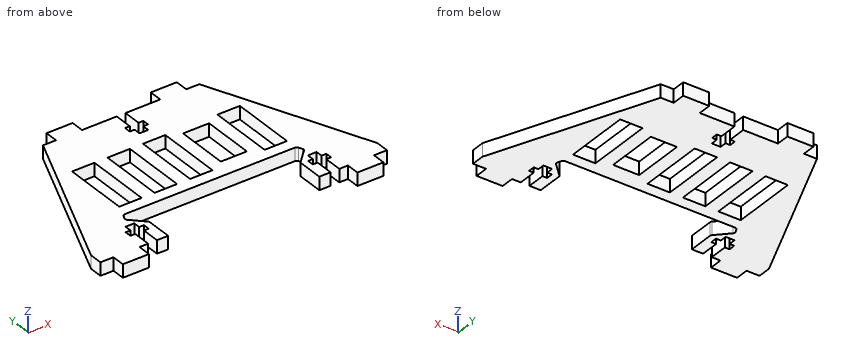
```python
from build123d import *

# Parameters (mm, degrees)
SKETCH1_W               = 139.7
SKETCH1_H               = 82.55
BOSS_EXTRUDE1_DEPTH     = 6.35
SKETCH2_W               = 12.7
SKETCH2_H               = 6.35
BOSS_EXTRUDE2_DEPTH     = 6.35
CUT_EXTRUDE1_DEPTH      = 6.35
CUT_EXTRUDE8_DEPTH      = 6.35
CUT_EXTRUDE2_DEPTH      = 6.35
CUT_EXTRUDE9_DEPTH      = 85.77904001
CUT_EXTRUDE9_DEPTH_BACK = 85.77904001
FILLET1_R               = 1.27
SKETCH9_W               = 10.922
SKETCH9_H               = 31.75
SKETCH9_W_2             = 12.7
SKETCH9_H_2             = 25.4
CUT_EXTRUDE10_DEPTH     = 6.35


with BuildPart() as part:
    # Sketch1 → Boss-Extrude1 (new body)
    with BuildSketch(Plane.XY):
        Rectangle(SKETCH1_W, SKETCH1_H)
    extrude(amount=BOSS_EXTRUDE1_DEPTH)

    # Sketch2 → Boss-Extrude2 (add)
    with BuildSketch(Plane(origin=(0, 0, 0), x_dir=(-1, 0, 0), z_dir=(0, 0, -1))):
        with Locations((-57.15, -44.45)):
            Rectangle(SKETCH2_W, SKETCH2_H)
        with Locations((-25.4, 44.45)):
            Rectangle(SKETCH2_W, SKETCH2_H)
    boss_extrude2 = extrude(amount=-BOSS_EXTRUDE2_DEPTH)

    # Sketch3 → Cut-Extrude1 (cut)
    with BuildSketch(Plane(origin=(0, 0, 0), x_dir=(-1, 0, 0), z_dir=(0, 0, -1))):
        Polygon((-46.5836, -41.275), (-46.5836, -32.512), (-48.895, -32.512), (-48.895, -29.337), (-46.5836, -29.337), (-46.5836, -26.035), (-42.3164, -26.035), (-42.3164, -29.337), (-40.005, -29.337), (-40.005, -32.512), (-42.3164, -32.512), (-42.3164, -41.275), align=None)
    cut_extrude1 = extrude(amount=-CUT_EXTRUDE1_DEPTH, mode=Mode.SUBTRACT)

    # Sketch7 → Cut-Extrude8 (cut)
    with BuildSketch(Plane(origin=(0, 0, 0), x_dir=(-1, 0, 0), z_dir=(0, 0, -1))):
        Polygon((-38.1, 41.275), (-69.85, -34.925), (-69.85, 41.275), align=None)
    cut_extrude8 = extrude(amount=-CUT_EXTRUDE8_DEPTH, mode=Mode.SUBTRACT)

    # Mirror2: Boss-Extrude2, Cut-Extrude8 across plane
    add(boss_extrude2.mirror(Plane(origin=(0, 0, 0), x_dir=(0, 0, 1), z_dir=(1, 0, 0))))
    add(cut_extrude8.mirror(Plane(origin=(0, 0, 0), x_dir=(0, 0, 1), z_dir=(1, 0, 0))), mode=Mode.SUBTRACT)

    # Mirror4: Cut-Extrude1 across plane
    add(cut_extrude1.mirror(Plane(origin=(0, 0, 0), x_dir=(0, 0, 1), z_dir=(1, 0, 0))), mode=Mode.SUBTRACT)

    # Sketch4 → Cut-Extrude2 (cut)
    with BuildSketch(Plane(origin=(0, 0, 0), x_dir=(-1, 0, 0), z_dir=(0, 0, -1))):
        Polygon((2.1336, 41.275), (-2.1336, 41.275), (-2.1336, 32.512), (-4.445, 32.512), (-4.445, 29.337), (-2.1336, 29.337), (-2.1336, 26.035), (2.1336, 26.035), (2.1336, 29.337), (4.445, 29.337), (4.445, 32.512), (2.1336, 32.512), align=None)
    extrude(amount=-CUT_EXTRUDE2_DEPTH, mode=Mode.SUBTRACT)

    # Sketch8 → Cut-Extrude9 (cut, two sides: drawn at the far end of the back side and taken through both)
    with BuildSketch(Plane.XY.offset(6.35).offset(-CUT_EXTRUDE9_DEPTH_BACK)):
        Polygon((-36.83, -28.575), (-43.702941176, -21.702058824), (-42.333333333, -18.415), (42.333333333, -18.415), (43.702941176, -21.702058824), (36.83, -28.575), (36.83, -41.275), (-36.83, -41.275), align=None)
    extrude(amount=CUT_EXTRUDE9_DEPTH + CUT_EXTRUDE9_DEPTH_BACK, mode=Mode.SUBTRACT)

    # Fillet1
    fillet1_edges = [part.edges().sort_by_distance(p)[0] for p in [
        (-36.83, -28.575, 3.175),
        (-43.702941176, -21.702058824, 3.175),
        (-42.333333333, -18.415, 3.175),
        (42.333333333, -18.415, 3.175),
        (43.702941176, -21.702058824, 3.175),
        (36.83, -28.575, 3.175),
    ]]
    fillet(fillet1_edges, radius=FILLET1_R)

    # Sketch9 → Cut-Extrude10 (cut)
    with BuildSketch(Plane.XY.offset(6.35)):
        with Locations((0, 3.175)):
            Rectangle(SKETCH9_W, SKETCH9_H)
        with Locations((-34.544, 3.175)):
            Rectangle(SKETCH9_W, SKETCH9_H)
        with Locations((-17.272, 3.175)):
            Rectangle(SKETCH9_W, SKETCH9_H)
        with Locations((36.322, 3.175)):
            Rectangle(SKETCH9_W, SKETCH9_H)
        with Locations((18.161, 3.175)):
            Rectangle(SKETCH9_W_2, SKETCH9_H_2)
    extrude(amount=-CUT_EXTRUDE10_DEPTH, mode=Mode.SUBTRACT)


solid = part.part
```
Source: CAD feature listing. Evaluate the final solid. Frame: model axes, mm. Coordinates: 2 decimals unless noted, no trailing zeros. Write each loop counter-clockwise with the first axis right and the second up, starting at its lowest first coordinate (ties: lowest second). Pieces come first, ordered by that corner, then holes. Notation, with made-up numbers: M 62,-7.5 L 106,-7.5 A22 ccw 106,21.5 Z; hole C 70,32.5 d7. An arc over 180 degrees is marked long. Answer as a JSON object with one key per item and string values.
1. Ray query, L1, parallel to X at y = -35.5, z = 0.5; L2, parallel to Y at x = 2.5, z = 5.5 (3 decimals); L3, parallel to Y at x = -2, z = 0.75 (3 decimals). Return the intervals inside material, ascending.
Evaluation:
{"L1": "-69.85 to -46.58, -42.32 to -36.83, 36.83 to 42.32, 46.58 to 69.85", "L2": "-18.415 to -12.7, 19.05 to 29.337, 32.512 to 41.275", "L3": "-18.415 to -12.7, 19.05 to 26.035"}
2. Contact query for flat-ended pins moving along their axis: P1, Ø1, axis at y = 27, z = 4.5, coming from the +X side; P2, Ø1.9, axis at y = 0, z = 4, coming from the +X side; P3, Ø3, axis at x = 20.5, z = 4, coming from the -Y side (3 decimals). Output: stop coordinate, or through.
Evaluation:
{"P1": "x = 44.26", "P2": "x = 55.69", "P3": "y = -18.415"}
3. Cut plane D-D on x = 17.5. Output: boundary loops of the cut face in (y, z) (3 decimals).
Evaluation:
{"outline": "M -18.415,0 L -9.525,0 L -9.525,6.35 L -18.415,6.35 Z; M 15.875,0 L 41.275,0 L 41.275,6.35 L 15.875,6.35 Z"}
4. Cut plane A-A on x = 34.5. Output: boundary loops of the cut face in (y, z) (3 decimals).
Evaluation:
{"outline": "M -18.415,0 L -12.7,0 L -12.7,6.35 L -18.415,6.35 Z; M 19.05,0 L 41.275,0 L 41.275,6.35 L 19.05,6.35 Z"}
5. Cut plane C-C on y = 2. Output: boundary loops of the cut face in (x, z) (3 decimals), plus the area to 3 significant figures.
Evaluation:
{"outline": "M -54.465,0 L -40.005,0 L -40.005,6.35 L -54.465,6.35 Z; M -29.083,0 L -22.733,0 L -22.733,6.35 L -29.083,6.35 Z; M -11.811,0 L -5.461,0 L -5.461,6.35 L -11.811,6.35 Z; M 5.461,0 L 11.811,0 L 11.811,6.35 L 5.461,6.35 Z; M 24.511,0 L 30.861,0 L 30.861,6.35 L 24.511,6.35 Z; M 41.783,0 L 54.465,0 L 54.465,6.35 L 41.783,6.35 Z", "area": "334 mm^2"}
6. Cut plane B-B on y = 17.5. Output: boundary loops of the cut face in (x, z) (3 decimals), plus the area to 3 significant figures.
Evaluation:
{"outline": "M -48.006,0 L -40.005,0 L -40.005,6.35 L -48.006,6.35 Z; M -29.083,0 L -22.733,0 L -22.733,6.35 L -29.083,6.35 Z; M -11.811,0 L -5.461,0 L -5.461,6.35 L -11.811,6.35 Z; M 5.461,0 L 30.861,0 L 30.861,6.35 L 5.461,6.35 Z; M 41.783,0 L 48.006,0 L 48.006,6.35 L 41.783,6.35 Z", "area": "332 mm^2"}
